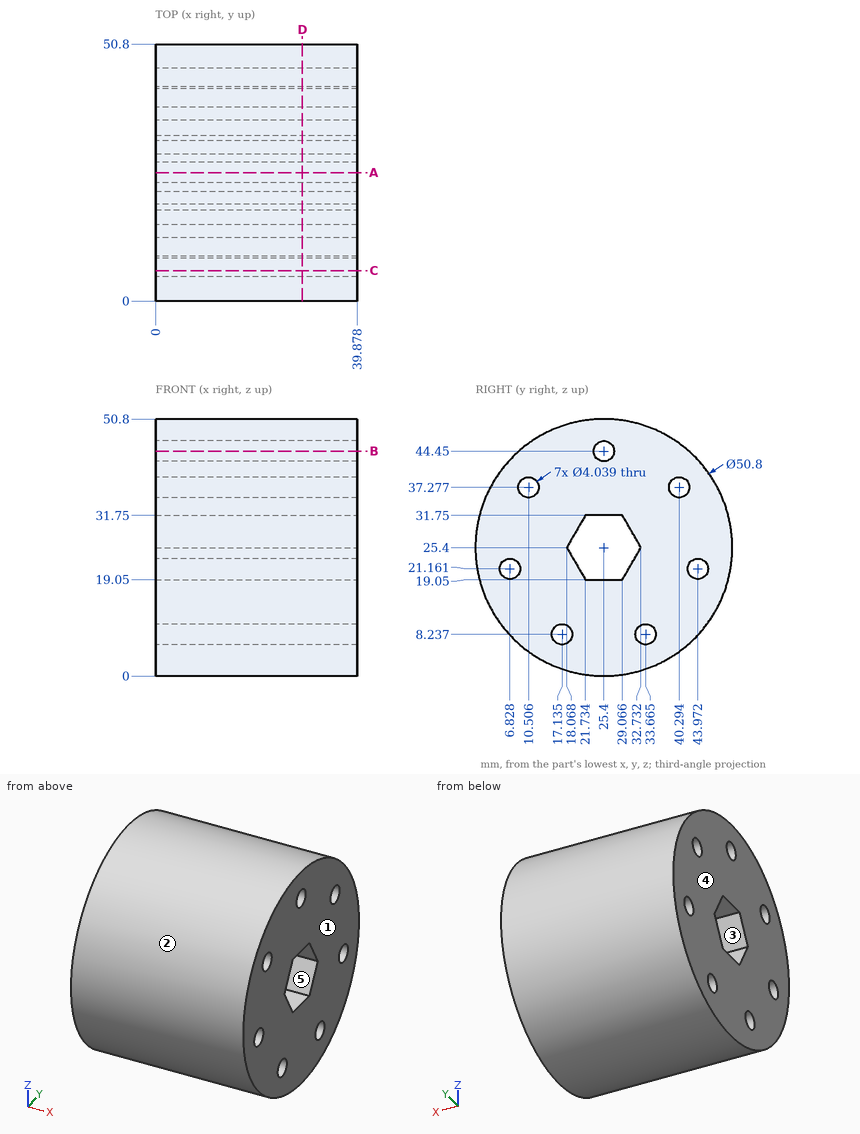
Geometry check sheet. Reference: drawing and pictorial views, mm from the part's lowest x, y, z. A direction names the side the tool comes from. Coordinates: 2 decimals unless noted, no trailing zeros. Loops run counter-clockwise (first coordinate to the right, second up) from the corner with the lowest first, then second, coordinate; pieces in that order, holes last.
1) Sectioned sample at C-C (y = 6). Record the boundary of the cut face in (x, z) (1 decimal), and give its area (3 significant figures).
2) Release check for a two-part mould opening along Y. For the marked faces 1, 2 and 3 record: released by +Y, released by -Y, zero draft, split by the parting line, or undercut.
3) Sectioned sample at D-D (x = 29). Count the separate pieces of the cut face and the enclosed holes in it, and give its area (3 significant figures).
4) Material ranges on probe 1 along Z at (x, y) = (30.5, 25.4); probe 2 along Y at (x, z) = (26.5, 20.5) (1 decimal); probe 3 along Y at (x, z) = (29.5, 37.5) (1 decimal), recorded low to high.
5) Gauge pin test, flat ends, axial feed: pin 1 (5 mm diameter, centred on x = 22, y = 25.5, fed in from +Z); pin 2 (2 mm diameter, centred on x = 18, y = 15, fed in from +Z); pin 3 (3 mm diameter, centred on x = 32.5, y = 29, fed in from -Z). Record the tip position at first contact, or that the pin passes through.
6) Sectioned sample at A-A (y = 25.4). Record the boundary of the cut face in (x, z).
7) Sectioned sample at B-B (z = 44.45). Record the boundary of the cut face in (x, y), and give its area (3 significant figures).
8) Access from +Z, -Z, +X, -X, +Y, -Y to the whole of each face (thin tool, end or side, straight path). Record for the marked faces 4 and 5.
Check sheet entries:
1. outline: (0, 9) - (39.9, 9) - (39.9, 19.3) - (0, 19.3) - close; (0, 23) - (39.9, 23) - (39.9, 41.8) - (0, 41.8) - close
1. area: 1,160 mm2
2. face 1: zero draft
2. face 2: split by the parting line
2. face 3: undercut
3. separate pieces: 1
3. enclosed holes: 8
3. area: 1,800 mm2
4. probe 1: z = 0 to 19.05, 31.75 to 42.43, 46.47 to 50.8
4. probe 2: y = 0.5 to 4.9, 8.7 to 20.9, 29.9 to 42.1, 45.9 to 50.3
4. probe 3: y = 3.1 to 8.5, 12.5 to 38.3, 42.3 to 47.7
5. pin 1: stops at z = 50.8
5. pin 2: stops at z = 49
5. pin 3: stops at z = 0.09
6. outline: (0, 0) - (39.88, 0) - (39.88, 19.05) - (0, 19.05) - close; (0, 31.75) - (39.88, 31.75) - (39.88, 42.43) - (0, 42.43) - close; (0, 46.47) - (39.88, 46.47) - (39.88, 50.8) - (0, 50.8) - close
7. outline: (0, 8.6) - (39.88, 8.6) - (39.88, 23.38) - (0, 23.38) - close; (0, 27.42) - (39.88, 27.42) - (39.88, 42.2) - (0, 42.2) - close
7. area: 1,180 mm2
8. face 4: +Z, -Z, -X, +Y, -Y
8. face 5: +X, -X
